Can you work these out from the drawing? Everything is in mm from the part's minimum corner. A direction names the side the tool comes from. Round coordinates to 2 decimals unless told otherwise and drop trailing zeros. Write each loop counter-clockwise with the first axis right and the second up, starting at its lowest first coordinate (ties: lowest second). Pieces come first, ordered by that corner, then holes. Notation, with made-up numbers: M 84,2 L 89,2 A34 ccw 89,38 Z; hole C -8,55.5 d2. An arc over 180 degrees is marked long. Answer in a Markdown table with one row per item. Add a question column.
(1) Suppose I cut it at C-C, the plane x = 35. Write out the boundary of the cut face in (y, z).
(2) Suppose I cut it at A-A, the plane y = 1. Count the separate pieces of the cut face and the enclosed holes in it, then the cut area to 3 significant figures.
(3) Suppose I cut it at B-B, the plane z = 35. Write out the boundary of the cut face in (x, y), then the cut area to 3 significant figures.
(4) I'm going to push flat-ended pins straight in: pin 1 (3 mm diameter, centred on x = 41.5, z = 58, fed in from +Y); pin 2 (2 mm diameter, centred on x = 13.5, y = 3.5, fed in from +Z). Where does each tip first touch, or does it pass through?
(5) If we mould it in two halves opening along Z, with no side actions, what happens to the marked faces 1 and 2? For each: released by +Z, released by -Z, zero draft, split by the parting line, or undercut.
(6) For the marked faces 3 and 4, which set-ups out of +Z, -Z, +X, -X, +Y, -Y let a thin tool reach every point of the face, with its end or its side?
(7) If I drill on probe 1 along X at (y, z) = (2.35, 35); probe 2 along Z at (x, y) = (34, 2.75) (1 decimal); probe 3 along Y at (x, z) = (12.5, 22), over which ranges is the centre line in solid material (lowest first)?
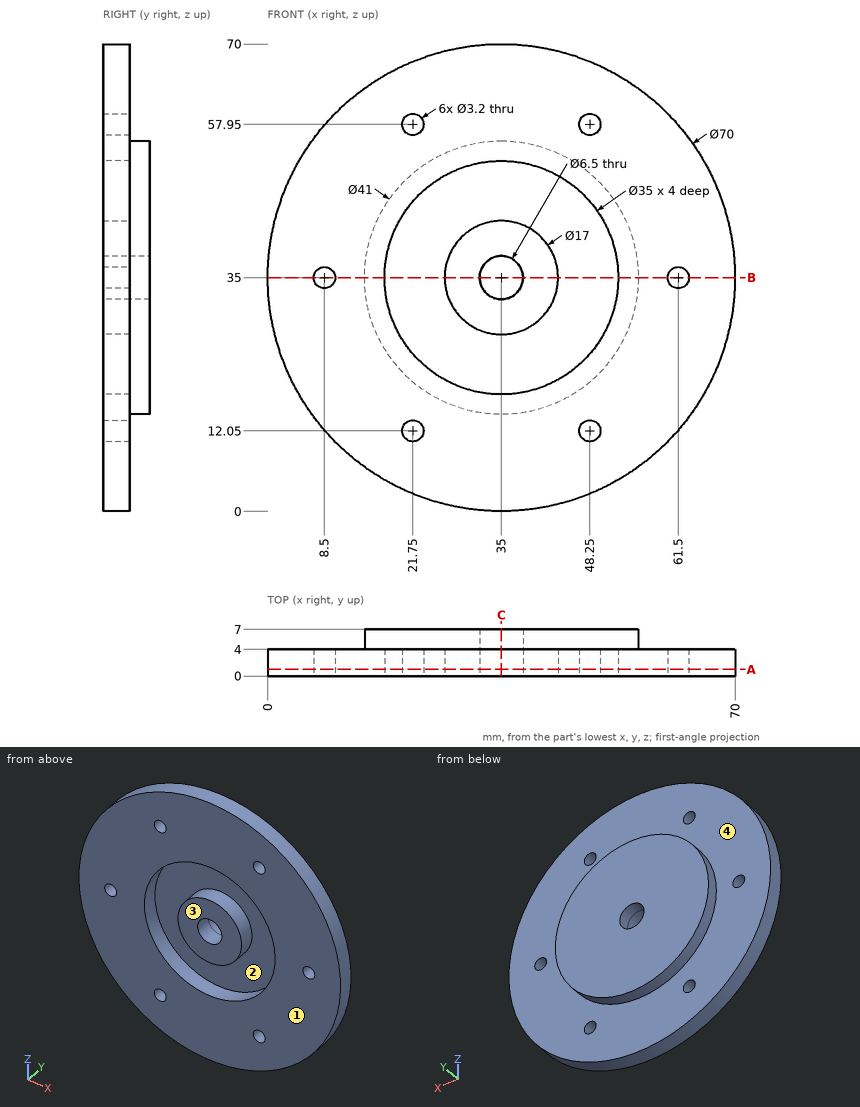
Calculated:
| question | item | result |
|---|---|---|
| 1 | outline | M 0,0 L 4,0 L 4,14.5 L 7,14.5 L 7,31.75 L 0,31.75 L 0,26.5 L 4,26.5 L 4,17.5 L 0,17.5 Z; M 0,38.25 L 7,38.25 L 7,55.5 L 4,55.5 L 4,70 L 0,70 L 0,52.5 L 4,52.5 L 4,43.5 L 0,43.5 Z |
| 2 | separate pieces | 2 |
| 2 | enclosed holes | 8 |
| 2 | area | 3,030 mm² |
| 3 | outline | M 0,0 L 6.9,0 L 6.9,4 L 0,4 Z; M 10.1,0 L 17.5,0 L 17.5,4 L 26.5,4 L 26.5,0 L 31.75,0 L 31.75,7 L 14.5,7 L 14.5,4 L 10.1,4 Z; M 38.25,0 L 43.5,0 L 43.5,4 L 52.5,4 L 52.5,0 L 59.9,0 L 59.9,4 L 55.5,4 L 55.5,7 L 38.25,7 Z; M 63.1,0 L 70,0 L 70,4 L 63.1,4 Z |
| 3 | area | 260 mm² |
| 4 | pin 1 | y = 4 |
| 4 | pin 2 | z = 63.37 |
| 5 | face 1 | zero draft |
| 5 | face 2 | undercut |
| 6 | face 3 | +Z, -Z, +X, -X, -Y |
| 6 | face 4 | +Y |
| 7 | probe 1 | 0 to 6.9, 10.1 to 17.5, 26.5 to 31.75, 38.25 to 43.5, 52.5 to 59.9, 63.1 to 70 |
| 7 | probe 2 | 0 to 17.5, 26.6 to 31.9, 38.1 to 43.4, 52.5 to 70 |
| 7 | probe 3 | 0 to 4 |
